Read the model definition and answer for the solid it produces. Units are mm, in the model's axes. A direction names the side the tool comes from. Coordinates: 2 decimals unless noted, no trailing zeros. Loops run counter-clockwise (first coordinate to the right, second up) from the corner with the lowest first, then second, coordinate; pieces in that order, holes last. Notation, with made-up numbers: (-9, -2.75) -> (34, -2.75) arc R9 cw to (34, 3.25) -> close; hole circle Ø9 at (47.5, -4). An arc over 180 degrees is marked (long way). Answer as CSV lines item,"result".
```python
from build123d import *

# Parameters (mm, degrees)
BASE_FLANGE1_DEPTH = 158.75
SKETCH8_R          = 2.4892
SKETCH8_W          = 25.4
SKETCH8_H          = 82.55
CUT_EXTRUDE1_DEPTH = 327.455070335
CUT_EXTRUDE3_START = 134.703841816
CUT_EXTRUDE3_DEPTH = 3.175


# Read off the part's stored shape, not the designer's step: Cut-Extrude3
# Sheet-metal steps are written as plain solids
with BuildPart() as part:
    # Sketch1 → Base-Flange1 (new, symmetric)
    with BuildSketch(Plane.XY):
        with BuildLine():
            Line((-80.82230509, 80.82230509), (-0.238063608, 0.238063608))
            ThreePointArc((-0.238063608, 0.238063608), (0.02562769, 0.061870716), (0.336672783, 0))
            Line((0.336672783, 0), (190.163327217, 0))
            ThreePointArc((190.163327217, 0), (190.47437231, 0.061870716), (190.738063608, 0.238063608))
            Line((190.738063608, 0.238063608), (271.32230509, 80.82230509))
            Line((271.32230509, 80.82230509), (273.56736912, 78.577241059))
            Line((273.56736912, 78.577241059), (192.983127639, -2.007000422))
            ThreePointArc((192.983127639, -2.007000422), (191.689392208, -2.8714468), (190.163327217, -3.175))
            Line((190.163327217, -3.175), (0.336672783, -3.175))
            ThreePointArc((0.336672783, -3.175), (-1.189392208, -2.8714468), (-2.483127639, -2.007000422))
            Line((-2.483127639, -2.007000422), (-83.06736912, 78.577241059))
            Line((-83.06736912, 78.577241059), (-80.82230509, 80.82230509))
        make_face()
    extrude(amount=BASE_FLANGE1_DEPTH, both=True)

    # Sketch8 → Cut-Extrude1 (cut, through all)
    with BuildSketch(Plane(origin=(0, 0, 0), x_dir=(1, 0, 0), z_dir=(0, 1, 0))):
        with Locations(Location((60.3885, 146.05, 0), (0, 0, 270))):
            Circle(SKETCH8_R)
        with Locations(Location((130.1115, 146.05, 0), (0, 0, 270))):
            Circle(SKETCH8_R)
        with Locations((60.3885, 92.075)):
            Rectangle(SKETCH8_W, SKETCH8_H)
        with Locations((130.1115, 92.075)):
            Rectangle(SKETCH8_W, SKETCH8_H)
    extrude(amount=-CUT_EXTRUDE1_DEPTH, mode=Mode.SUBTRACT)

    # Cut-Extrude3 outline → Cut-Extrude3 (cut)
    with BuildSketch(Plane(origin=(0, 0, 0), x_dir=(0.7071067811865472, 0.7071067811865479, 0), z_dir=(0.7071067811865479, -0.707106781186547, 0)).offset(CUT_EXTRUDE3_START)):
        with BuildLine():
            add(Edge.make_bspline(
                [(151.754493433, -150.8125), (145.019301342, -150.8125), (145.019301342, -146.05), (145.019301342, -141.2875), (151.754493433, -141.2875)],
                knots=[4.71238898, 4.71238898, 4.71238898, 6.283185307, 6.283185307, 7.853981634, 7.853981634, 7.853981634], degree=2, weights=[1, 0.707106781, 1, 0.707106781, 1]))
            Line((151.754493433, -150.8125), (154.929493433, -150.8125))
            add(Edge.make_bspline(
                [(154.929493433, -141.2875), (161.664685524, -141.2875), (161.664685524, -146.05), (161.664685524, -150.8125), (154.929493433, -150.8125)],
                knots=[1.570796327, 1.570796327, 1.570796327, 3.141592654, 3.141592654, 4.71238898, 4.71238898, 4.71238898], degree=2, weights=[1, 0.707106781, 1, 0.707106781, 1]))
            Line((154.929493433, -141.2875), (151.754493433, -141.2875))
        make_face()
    extrude(amount=CUT_EXTRUDE3_DEPTH, mode=Mode.SUBTRACT)


solid = part.part
```
Q1. A cutting plane is placed at B-B, the plane y = 72. Write down the section's boundary in (x, z).
Results:
outline,"(-76.49, -158.75) -> (-72, -158.75) -> (-72, 158.75) -> (-76.49, 158.75) -> close; (262.5, -158.75) -> (266.99, -158.75) -> (266.99, 158.75) -> (262.5, 158.75) -> close"
Q2. A cutting plane is placed at D-D, the plane x = 102. Write down the section's boundary in (y, z) (3 decimals).
Results:
outline,"(-3.175, -158.75) -> (0, -158.75) -> (0, 158.75) -> (-3.175, 158.75) -> close"
Q3. Given pin 1 Ø3.5 at (y, z) = (-2, -79.5) entering from +X; pin 2 Ø3.5 at (y, z) = (-1.5, -100) entering from -X; pin 3 Ø2 at (y, z) = (62.5, 42) entering from -X, each flat-ended and moving along its own axis, determine where each tip first touches the part or whether it passes through.
Results:
pin 1,"stops at x = 194.74"
pin 2,"stops at x = -4.74"
pin 3,"stops at x = -67.99"
Q4. For a pull along X with two mould halves and no side action, classify faces 1 (the face through (94, 0, 2)), 2 (the face through (97, -3.175, 2)), 3 (the face through (-42.21, 37.72, 2.22)) as pulls with the +X half, pulls with the -X half, needs draft (parallel to the pull), parting line crosses it, or undercut.
Results:
face 1,"undercut"
face 2,"needs draft"
face 3,"pulls with the -X half"
Q5. For faces 4 (the face through (109, -1, -158.75)), 5 (the face through (-41, 41, 2)), determine the directions among +Z, -Z, +X, -X, +Y, -Y from which every point of the face is accessible in a straight line to the end or side of a thin tool.
Results:
face 4,"-Z, +X, -X, +Y, -Y"
face 5,"+Z, -Z, +Y"
Q6. A cutting plane is placed at A-A, the plane z = -82.5. Write down the section's boundary in (x, y) (1 decimal), and give its area (3 significant figures).
Results:
outline,"(-83.1, 78.6) -> (-2.5, -2) arc R4 ccw to (0.3, -3.2) -> (47.7, -3.2) -> (47.7, 0) -> (0.3, 0) arc R0.8 cw to (-0.2, 0.2) -> (-80.8, 80.8) -> close; (73.1, -3.2) -> (117.4, -3.2) -> (117.4, 0) -> (73.1, 0) -> close; (142.8, -3.2) -> (190.2, -3.2) arc R4 ccw to (193, -2) -> (273.6, 78.6) -> (271.3, 80.8) -> (190.7, 0.2) arc R0.8 cw to (190.2, 0) -> (142.8, 0) -> close"
area,"1,180 mm²"
Q7. Find the intervals of material crossed by probe 1 along X at (y, z) = (-1, -146); probe 2 along X at (y, z) = (-1.75, -146.05); probe 3 along Y at (x, z) = (127, 119) (3 decimals), in increasing order. Write a range as [from, to].
Results:
probe 1,"x = [-3.49, 57.9], [62.88, 127.62], [132.6, 193.99]"
probe 2,"x = [-2.74, 57.9], [62.88, 127.62], [132.6, 193.24]"
probe 3,"y = [-3.175, 0]"
Q8. A cutting plane is placed at C-C, the plane z = -2. Write down the section's boundary in (x, y) (3 decimals).
Results:
outline,"(-83.067, 78.577) -> (-2.483, -2.007) arc R3.988 ccw to (0.337, -3.175) -> (190.163, -3.175) arc R3.988 ccw to (192.983, -2.007) -> (273.567, 78.577) -> (271.322, 80.822) -> (190.738, 0.238) arc R0.813 cw to (190.163, 0) -> (0.337, 0) arc R0.813 cw to (-0.238, 0.238) -> (-80.822, 80.822) -> close"
